CAD build for the part. Positions are in the model's coordinates, mm. A direction names the side the tool comes from. Coordinates: 2 decimals unless noted, no trailing zeros. Write each loop counter-clockwise with the first axis right and the second up, starting at its lowest first coordinate (ties: lowest second). Pieces come first, ordered by that corner, then holes.
```python
from build123d import *

# Parameters (mm, degrees)
SKETCH_1_W          = 500
SKETCH_1_H          = 240
EXTRUDE_1_DEPTH     = 10
SHELL_1_T           = -8
EXTRUDE_2_DEPTH     = 20
SKETCH_9_R          = 1.65
CUT_EXTRUDE_1_DEPTH = 10


with BuildPart() as part:
    # 草圖1 → 填料-伸長1 (new body)
    with BuildSketch(Plane.XY):
        Rectangle(SKETCH_1_W, SKETCH_1_H)
    extrude(amount=EXTRUDE_1_DEPTH)

    # 薄殼1
    shell_1_openings = [part.faces().sort_by_distance(p)[0] for p in [
        (0, 0, 10),
    ]]
    offset(amount=SHELL_1_T, openings=shell_1_openings, kind=Kind.INTERSECTION)

    # 草圖2 → 填料-伸長2 (add)
    with BuildSketch(Plane(origin=(0, 0, 0), x_dir=(-1, 0, 0), z_dir=(0, 0, -1))):
        with BuildLine():
            Line((-30, -40), (30, -40))
            ThreePointArc((30, -40), (37.071067812, -37.071067812), (40, -30))
            Line((40, -30), (40, 30))
            ThreePointArc((40, 30), (37.071067812, 37.071067812), (30, 40))
            Line((30, 40), (-30, 40))
            ThreePointArc((-30, 40), (-37.071067812, 37.071067812), (-40, 30))
            Line((-40, 30), (-40, -30))
            ThreePointArc((-40, -30), (-37.071067812, -37.071067812), (-30, -40))
        make_face()
    extrude(amount=EXTRUDE_2_DEPTH)

    # 草圖9 → 除料-伸長1 (cut)
    with BuildSketch(Plane(origin=(0, 0, -20), x_dir=(-1, 0, 0), z_dir=(0, 0, -1))):
        Circle(SKETCH_9_R)
    extrude(amount=-CUT_EXTRUDE_1_DEPTH, mode=Mode.SUBTRACT)


solid = part.part
```
Item 1: Wall check: line 1 along Y through (x, z) = (0, -15); line 2 along Z through (x, y) = (-35.5, -62); line 3 along Y through (x, z) = (-17.5, -13.5). Give the ranges that are in metal, low to high.
Item 2: Flat gauge pins, fed straight in: pin 1 Ø10 at (x, z) = (-13, -12) entering from +Y; pin 2 Ø2 at (x, y) = (0, 0) entering from +Z; pin 3 Ø6 at (y, z) = (-7, -8) entering from -X; pin 4 Ø10 at (y, z) = (5.5, -2) entering from +X. Where does each tip first touch, or does it go through?
Item 3: Which spindle directions (+Z, -Z, +X, -X, +Y, -Y) get a long thin tool onto all of the face, cutting with end or side? Do faces 4 (the flat face through (40, 0, -10)), 5 (the cylindrical face through (-36.99, -37.15, -9.86)), 6 (the cylindrical face through (37.15, -36.99, -9.86)), 7 (the flat face through (0, -40, -10)), 8 (the flat face through (-40, 0, -10)). Say none if no direction does.
Item 4: Saw through at B-B, the plane x = -168.5. Write the cut outline in (y, z), and give its area (3 significant figures).
Item 5: Saw through at A-A, the plane y = -6.5. Write the cut outline in (x, z).
Item 6: Saw through at C-C, the plane y = 101.5. Write the cut outline in (x, z), and give its area (3 significant figures).
Item 7: Two-plate mould, pull along Y, no slides. Class faces 1 (the flat face through (-3, 2, 8)), 2 (the flat face through (-3, 55, 0)), 3 (the flat face through (-3, 120, 5)): +Y half, -Y half, draft (parallel to the pull), parting line (faces both ways), or undercut.
Working result:
1. line 1: y = -40 to -1.65, 1.65 to 40
1. line 2: z = 0 to 8
1. line 3: y = -40 to 40
2. pin 1: stops at y = 40
2. pin 2: stops at z = 8
2. pin 3: stops at x = -40
2. pin 4: stops at x = 250
3. face 4: -Z, +X, +Y, -Y
3. face 5: -Z, -X, -Y
3. face 6: -Z, +X, -Y
3. face 7: -Z, +X, -X, -Y
3. face 8: -Z, -X, +Y, -Y
4. outline: (-120, 0) - (120, 0) - (120, 10) - (112, 10) - (112, 8) - (-112, 8) - (-112, 10) - (-120, 10) - close
4. area: 1,950 mm2
5. outline: (-250, 0) - (-40, 0) - (-40, -20) - (40, -20) - (40, 0) - (250, 0) - (250, 10) - (242, 10) - (242, 8) - (-242, 8) - (-242, 10) - (-250, 10) - close
6. outline: (-250, 0) - (250, 0) - (250, 10) - (242, 10) - (242, 8) - (-242, 8) - (-242, 10) - (-250, 10) - close
6. area: 4,030 mm2
7. face 1: undercut
7. face 2: draft
7. face 3: +Y half
